Solid Edge part; units mm, degrees
sketch "Sketch1" plane through (0, 0, 293.0295) normal (0, 0, 1) x (1, 0, 0)
  line L0 (175.4, 73.6281) -> (175.4, -6.3719)
  line L1 (175.4, -6.3719) -> (174.6, -6.3719)
  line L2 (174.6, 73.6281) -> (174.6, -6.3719)
  line L3 (174.6, 73.6281) -> (175.4, 73.6281)
extrude "Protrusion1" add sketch "Sketch1" along normal blind 18
sketch "Sketch2" plane through (174.6, 56.2359, 300.5295) normal (-1, 0, 0) x (0, 0, 1)
  circle A0 centre (4.5, 11.3922) radius 2
  line L0 (10.5, -70.6078) -> (0.5, -70.6078)
  line L1 (0.5, -70.6078) -> (0.5, -0.6078)
  line L2 (0.5, -0.6078) -> (10.5, -0.6078)
  line L3 (10.5, -0.6078) -> (10.5, -70.6078)
  dimension "D1" = 0.5
  dimension "D2" = 10.5
extrude "Cutout1" cut sketch "Sketch2" along normal through all and the other way through all
sketch "Sketch3" plane through (175.4, 33.6281, 302.0295) normal (1, 0, 0) x (0, 1, 0)
  line L0 (0, -9) -> (-15, -9)
  line L1 (-15, -9) -> (-15, -1)
  line L2 (-15, -1) -> (-0.1222, -1)
  line L3 (-0.1222, -1) -> (0, -9)
extrude "ExtrudedCutout_2" cut sketch "Sketch3" against normal blind 0.1
The model under review builds one solid part; all positions refer to its coordinate system, in mm. Round coordinates to 2 decimals unless told otherwise and drop trailing zeros. Write each loop counter-clockwise with the first axis right and the second up, starting at its lowest first coordinate (ties: lowest second). Pieces come first, ordered by that corner, then holes. Notation, with made-up numbers: (7, 3.5) - (26, 3.5) arc R11 ccw to (26, 9.5) - close; hole circle Ø1 at (-10.75, -18.5). An arc over 180 degrees is marked (long way). One line per item, written item: value. Start each with the question number.
1. Consider section C-C on y = 54. Write out the cut boundary in (x, z), and give its area (3 significant figures).
2. The part is to be moulded in two halves that separate along Y. For faces 1 (the face through (175.3, 26, 297)), 2 (the face through (174.994, 68.229, 306.937)), 3 (the face through (175.4, 58, 300)), say which applies: released by +Y, released by -Y, zero draft, split by the parting line, or undercut.
3. To check wall thickness, follow L1, parallel to Y at x = 175.2, z = 305.25; L2, parallel to Y at x = 175.2, z = 309; L3, parallel to Z at x = 174.8, y = 21.5. State the ranges of each line that lie inside material, in increasing order. Write a range as from..to.
4. Consider section A-A on x = 175. Write out the cut boundary in (y, z).
5. Consider section B-B on z = 294.75. Write out the cut boundary in (x, y).
6. Consider section D-D on z = 299.5. Write out the cut boundary in (x, y), and give its area (3 significant figures).
7. Clearance check with a flat-ended pin moving along its axis: P1, Ø3, axis at y = 67.63, z = 305.03, coming from the -X side. State where the tip first meets the part, or that it passes through.
Checks:
1. outline: (174.6, 293.03) - (175.4, 293.03) - (175.4, 301.03) - (174.6, 301.03) - close
1. area: 6.40 mm^2
2. face 1: undercut
2. face 2: undercut
2. face 3: zero draft
3. L1: y = 55.63..65.64, 69.62..73.63
3. L2: y = 55.63..73.63
3. L3: z = 293.03..301.03
4. outline: (-6.37, 293.03) - (73.63, 293.03) - (73.63, 311.03) - (55.63, 311.03) - (55.63, 301.03) - (-6.37, 301.03) - close; hole circle Ø4 at (67.63, 305.03)
5. outline: (174.6, -6.37) - (175.4, -6.37) - (175.4, 18.63) - (175.3, 18.63) - (175.3, 33.6) - (175.4, 33.6) - (175.4, 73.63) - (174.6, 73.63) - close
6. outline: (174.6, -6.37) - (175.4, -6.37) - (175.4, 18.63) - (175.3, 18.63) - (175.3, 33.53) - (175.4, 33.53) - (175.4, 73.63) - (174.6, 73.63) - close
6. area: 62.5 mm^2
7. P1: passes through
